Model file for the job. Use its own axes, mm. A direction names the side the tool comes from. Coordinates: 2 decimals unless noted, no trailing zeros. Write each loop counter-clockwise with the first axis right and the second up, starting at its lowest first coordinate (ties: lowest second). Pieces come first, ordered by that corner, then holes.
Q1. Band-saw the part on A-A, the plane y = 96. Write the cut outline in (x, z).
Q2. Band-saw the part on B-B, the plane z = 22.5. Write the cut outline in (x, y).
Q3. Band-saw the part on D-D, the plane y = 166.5. Write the cut outline in (x, z), plus the area to 3 significant figures.
Q4. Band-saw the part on C-C, the plane x = 0. State how many separate pieces and enclosed holes the cut face has, plus the area to 3 significant figures.
Q5. Pin check, flat tips, straight feed: P1, Ø1.5, axis at y = 134, z = 6.5, coming from the -X side; P2, Ø3, axis at x = -20.5, z = 30.5, coming from the +Y side; P3, Ø3, axis at x = -21.5, z = 19, coming from the -Y side; P4, Ø18, axis at x = 0, y = 0, coming from the -Z side. Stop position of each tip, or through.
Q6. Drill centre lines: probe 1 along Z at (x, y) = (10, 581.5); probe 2 along Y at (x, z) = (20.5, 12); probe 3 along Y at (x, z) = (2.5, 38). Where is each one in solid material? Low to high.
Q7. Which spindle directions (+Z, -Z, +X, -X, +Y, -Y) get a long thin tool onto all of the face, cutting with end or side? Do faces 5 (the cylindrical face through (-2.38, 422.42, 28.31)), 6 (the cylindrical face through (-0.605, -27.493, 2.465)), 7 (the flat face through (0, 290, 6)). Say none if no direction does.
Q8. Pull direction X, two halves, no side cores. Call faces 1 (the cylindrical face through (-1.302, 659.915, 2.465)), 2 (the flat face through (0, 330, 0)), 3 (the cylindrical face through (-0.594, 676.993, 52.465)), 4 (the flat face through (0, 433, 6)): released by +X, released by -X, zero draft, split by the parting line, or undercut.
from build123d import *

# Parameters (mm, degrees)
SKETCH1_R               = 10
BOSS_EXTRUDE2_DEPTH     = 5
BOSS_EXTRUDE3_DEPTH     = 55
BOSS_EXTRUDE4_START     = 50
SKETCH1_4_R             = 10
BOSS_EXTRUDE4_DEPTH     = 5
CUT_EXTRUDE1_DEPTH      = 682.432576538
CUT_EXTRUDE1_DEPTH_BACK = 682.432576538
SKETCH3_W               = 37
SKETCH3_H               = 564.316545641
SKETCH4_R               = 11
BOSS_EXTRUDE5_DEPTH     = 49


with BuildPart() as part:
    # Sketch1 → Boss-Extrude2 (new body)
    with BuildSketch(Plane.XY):
        with BuildLine():
            Line((27.00967764, 637.419067567), (27, 650))
            ThreePointArc((27, 650), (11.628325989, 674.367643191), (-16.983854422, 670.989251749))
            ThreePointArc((-16.983854422, 670.989251749), (-24.367643191, 661.628325989), (-27, 650))
            Line((-27, 650), (-27.00967764, 637.419067567))
            Line((-27.00967764, 637.419067567), (-17.00967764, 637.419067567))
            Line((-17.00967764, 637.419067567), (-17.490017949, 12.976666451))
            Line((-17.490017949, 12.976666451), (-27.490017949, 12.976666451))
            Line((-27.490017949, 12.976666451), (-27.5, 0))
            ThreePointArc((-27.5, 0), (0, -27.5), (27.5, 0))
            Line((27.5, 0), (27.490017949, 12.976666451))
            Line((27.490017949, 12.976666451), (17.490017949, 12.976666451))
            Line((17.490017949, 12.976666451), (17.00967764, 637.419067567))
            Line((17.00967764, 637.419067567), (27.00967764, 637.419067567))
        make_face()
        Circle(SKETCH1_R, mode=Mode.SUBTRACT)
        with Locations((0, 650)):
            Circle(SKETCH1_R, mode=Mode.SUBTRACT)
    extrude(amount=BOSS_EXTRUDE2_DEPTH)

    # Sketch1_3 → Boss-Extrude3 (add)
    with BuildSketch(Plane.XY):
        Polygon((27.490017949, 12.976666451), (27.00967764, 637.419067567), (17.00967764, 637.419067567), (17.490017949, 12.976666451), align=None)
        Polygon((-17.00967764, 637.419067567), (-27.00967764, 637.419067567), (-27.490017949, 12.976666451), (-17.490017949, 12.976666451), align=None)
    extrude(amount=BOSS_EXTRUDE3_DEPTH)

    # Sketch1_4 → Boss-Extrude4 (add)
    with BuildSketch(Plane.XY.offset(BOSS_EXTRUDE4_START)):
        with BuildLine():
            Line((27, 650), (27.5, 0))
            ThreePointArc((27.5, 0), (0, -27.5), (-27.5, 0))
            Line((-27.5, 0), (-27, 650))
            ThreePointArc((-27, 650), (0, 677), (27, 650))
        make_face()
        Circle(SKETCH1_4_R, mode=Mode.SUBTRACT)
        with Locations((0, 650)):
            Circle(SKETCH1_4_R, mode=Mode.SUBTRACT)
    extrude(amount=BOSS_EXTRUDE4_DEPTH)

    # Sketch3 → Cut-Extrude1 (cut, two sides: drawn at the far end of the back side and taken through both)
    with BuildSketch(Plane(origin=(27.499983728, 0.021153834, 0), x_dir=(0, 0, -1), z_dir=(0.9999997041421432, 0.0007692305416477979, 0)).offset(-CUT_EXTRUDE1_DEPTH_BACK)):
        with Locations((-27.5, 330.399690719)):
            Rectangle(SKETCH3_W, SKETCH3_H)
    extrude(amount=CUT_EXTRUDE1_DEPTH + CUT_EXTRUDE1_DEPTH_BACK, mode=Mode.SUBTRACT)

    # Sketch4 → Boss-Extrude5 (add)
    with BuildSketch(Plane.XY.offset(55)):
        with Locations((0, 569.255461643)):
            Circle(SKETCH4_R)
        with Locations((0, 433.161322259)):
            Circle(SKETCH4_R)
        with Locations((0, 290.166334704)):
            Circle(SKETCH4_R)
        with Locations((0, 141.938836299)):
            Circle(SKETCH4_R)
    extrude(amount=-BOSS_EXTRUDE5_DEPTH)


solid = part.part
Answer sheet:
1. outline: (-27.43, 0) - (27.43, 0) - (27.43, 9) - (17.43, 9) - (17.43, 5) - (-17.43, 5) - (-17.43, 9) - (-27.43, 9) - close; (-27.43, 46) - (-17.43, 46) - (-17.43, 50) - (17.43, 50) - (17.43, 46) - (27.43, 46) - (27.43, 55) - (-27.43, 55) - close
2. outline: (-27.49, 12.98) - (-17.49, 12.98) - (-17.46, 48.23) - (-27.46, 48.22) - close; (-27.03, 612.54) - (-17.03, 612.55) - (-17.01, 637.42) - (-27.01, 637.42) - close; circle Ø22 at (0, 141.94); circle Ø22 at (0, 290.17); circle Ø22 at (0, 433.16); circle Ø22 at (0, 569.26); (17.01, 637.42) - (17.03, 612.57) - (27.03, 612.58) - (27.01, 637.42) - close; (17.46, 48.25) - (17.49, 12.98) - (27.49, 12.98) - (27.46, 48.26) - close
3. outline: (-27.37, 0) - (27.37, 0) - (27.37, 9) - (17.37, 9) - (17.37, 5) - (-17.37, 5) - (-17.37, 9) - (-27.37, 9) - close; (-27.37, 46) - (-17.37, 46) - (-17.37, 50) - (17.37, 50) - (17.37, 46) - (27.37, 46) - (27.37, 55) - (-27.37, 55) - close
3. area: 707 mm2
4. separate pieces: 6
4. enclosed holes: 0
4. area: 10,500 mm2
5. P1: stops at x = -27.4
5. P2: stops at y = 637.42
5. P3: stops at y = 12.98
5. P4: passes through
6. probe 1: z = 0 to 5, 50 to 55
6. probe 2: y = 12.98 to 48.26, 612.57 to 637.42
6. probe 3: y = 131.23 to 152.65, 279.45 to 300.88, 422.45 to 443.87, 558.54 to 579.97
7. face 5: none
7. face 6: +Z, -Z, -Y
7. face 7: +Y, -Y
8. face 1: undercut
8. face 2: zero draft
8. face 3: split by the parting line
8. face 4: undercut
